Check sheet for the modelled part. Datum: model origin and axes. Units: mm. Face numbers are marked on the shaded views. A direction names the side the tool comes from. Give positions to 0.01 mm unless a question says otherwise; leave off trailing zeros. Order: outer loops, then holes, each group sorted by start corner. A loop starts at its lowest first (then second) coordinate and runs counter-clockwise, first axis right, second up.
Item 1: Sectioned sample at A-A on z = -4. Record the boundary of the cut face in (x, y), and give its area (3 significant figures).
Item 2: Sectioned sample at B-B on x = 0. Record the boundary of the cut face in (y, z).
Item 3: Gauge pin test, flat ends, axial feed: P1, Ø1.8, axis at x = 0, y = 5, coming from the +Z side; P2, Ø0.9, axis at x = -15, y = -3, coming from the -Z side; P3, Ø1.5, axis at y = 2.5, z = -1, coming from the -X side; P4, Ø1.8, axis at x = 15, y = -3, coming from the -Z side. Record the tip position at first contact, or that the pin passes through.
Item 4: Release check for a two-part mould opening along Y. For the marked faces 1, 2 and 3 record: released by +Y, released by -Y, zero draft, split by the parting line, or undercut.
Item 5: Sectioned sample at C-C on z = -2. Record the boundary of the cut face in (x, y), and give its area (3 significant figures).
Item 6: Access from +Z, -Z, +X, -X, +Y, -Y to the whole of each face (thin tool, end or side, straight path). Record for the marked faces 4, 5 and 6.
Item 7: Material ranges on line 1 along Y through (x, z) = (-15, -4.15); line 2 along X through (y, z) = (-3.25, -5.5); line 3 along Y through (x, z) = (15, -6.25), recorded low to high.
Item 8: Sectioned sample at D-D on y = 3. Record the boundary of the cut face in (x, z), and give its area (3 significant figures).
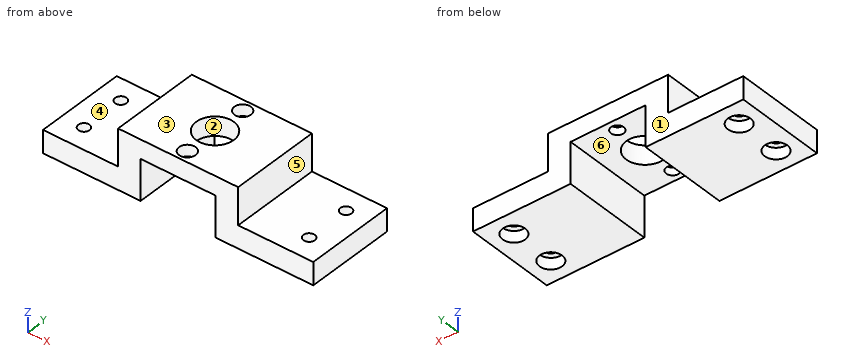
from build123d import *

# Parameters (mm, degrees)
SKETCH_1_W          = 10
SKETCH_1_H          = 12
SKETCH_1_R          = 0.85
SKETCH_1_R_2        = 2.5
EXTRUDE_1_DEPTH     = 1.25
CUT_EXTRUDE_START   = 1.25
SKETCH_1_6_R        = 1.1
CUT_EXTRUDE_1_DEPTH = 1.5
SKETCH_2_W          = 3
SKETCH_2_H          = 12
EXTRUDE_2_DEPTH     = 7.9
SKETCH_3_W          = 10
SKETCH_3_H          = 3
EXTRUDE_3_DEPTH     = 12
SKETCH_4_R          = 0.75
CUT_EXTRUDE_2_DEPTH = 21.552615405
SKETCH_4_3_R        = 1.5
CUT_EXTRUDE_3_DEPTH = 1.5


with BuildPart() as part:
    # 草图1 → 凸台-拉伸1 (new, symmetric)
    with BuildSketch(Plane.XY):
        Rectangle(SKETCH_1_W, SKETCH_1_H)
        with Locations((0, 4.5)):
            Circle(SKETCH_1_R, mode=Mode.SUBTRACT)
        with Locations((0, -4.5)):
            Circle(SKETCH_1_R, mode=Mode.SUBTRACT)
        Circle(SKETCH_1_R_2, mode=Mode.SUBTRACT)
    extrude(amount=EXTRUDE_1_DEPTH, both=True)

    # 草图1<6> → 切除-拉伸1 (cut)
    with BuildSketch(Plane.XY.offset(CUT_EXTRUDE_START)):
        with Locations((0, 4.5)):
            Circle(SKETCH_1_6_R)
        with Locations((0, -4.5)):
            Circle(SKETCH_1_6_R)
    extrude(amount=-CUT_EXTRUDE_1_DEPTH, mode=Mode.SUBTRACT)

    # 草图2 → 凸台-拉伸2 (add)
    with BuildSketch(Plane.XY.offset(1.25)):
        with Locations((6.5, 0)):
            Rectangle(SKETCH_2_W, SKETCH_2_H)
        with Locations((-6.5, 0)):
            Rectangle(SKETCH_2_W, SKETCH_2_H)
    extrude(amount=-EXTRUDE_2_DEPTH)

    # 草图3 → 凸台-拉伸3 (add)
    with BuildSketch(Plane(origin=(0, 6, 0), x_dir=(1, 0, 0), z_dir=(0, 1, 0))):
        with Locations((-13, 5.15)):
            Rectangle(SKETCH_3_W, SKETCH_3_H)
        with Locations((13, 5.15)):
            Rectangle(SKETCH_3_W, SKETCH_3_H)
    extrude(amount=-EXTRUDE_3_DEPTH)

    # 草图4 → 切除-拉伸2 (cut, through all)
    with BuildSketch(Plane(origin=(0, 0, -6.65), x_dir=(-1, 0, 0), z_dir=(0, 0, -1))):
        with Locations((15, -3)):
            Circle(SKETCH_4_R)
        with Locations((15, 3)):
            Circle(SKETCH_4_R)
        with Locations((-15, -3)):
            Circle(SKETCH_4_R)
        with Locations((-15, 3)):
            Circle(SKETCH_4_R)
    extrude(amount=-CUT_EXTRUDE_2_DEPTH, mode=Mode.SUBTRACT)

    # 草图4<3> → 切除-拉伸3 (cut)
    with BuildSketch(Plane(origin=(0, 0, -6.65), x_dir=(-1, 0, 0), z_dir=(0, 0, -1))):
        with Locations((15, 3)):
            Circle(SKETCH_4_3_R)
        with Locations((15, -3)):
            Circle(SKETCH_4_3_R)
        with Locations((-15, 3)):
            Circle(SKETCH_4_3_R)
        with Locations((-15, -3)):
            Circle(SKETCH_4_3_R)
    extrude(amount=-CUT_EXTRUDE_3_DEPTH, mode=Mode.SUBTRACT)


solid = part.part
Report:
1. outline: (-18, -6) - (-5, -6) - (-5, 6) - (-18, 6) - close; (5, -6) - (18, -6) - (18, 6) - (5, 6) - close; hole circle Ø1.5 at (-15, -3); hole circle Ø1.5 at (-15, 3); hole circle Ø1.5 at (15, -3); hole circle Ø1.5 at (15, 3)
1. area: 305 mm2
2. outline: (-6, -1.25) - (-5.35, -1.25) - (-5.35, -0.25) - (-5.6, -0.25) - (-5.6, 1.25) - (-6, 1.25) - close; (-3.65, -1.25) - (-2.5, -1.25) - (-2.5, 1.25) - (-3.4, 1.25) - (-3.4, -0.25) - (-3.65, -0.25) - close; (2.5, -1.25) - (3.65, -1.25) - (3.65, -0.25) - (3.4, -0.25) - (3.4, 1.25) - (2.5, 1.25) - close; (5.35, -1.25) - (6, -1.25) - (6, 1.25) - (5.6, 1.25) - (5.6, -0.25) - (5.35, -0.25) - close
3. P1: stops at z = 1.25
3. P2: passes through
3. P3: stops at x = -8
3. P4: stops at z = -5.15
4. face 1: released by +Y
4. face 2: undercut
4. face 3: zero draft
5. outline: (-8, -6) - (-5, -6) - (-5, 6) - (-8, 6) - close; (5, -6) - (8, -6) - (8, 6) - (5, 6) - close
5. area: 72.0 mm2
6. face 4: +Z, -X, +Y, -Y
6. face 5: +Z, +X, +Y, -Y
6. face 6: -Z, +Y, -Y
7. line 1: y = -6 to -3.75, -2.25 to 2.25, 3.75 to 6
7. line 2: x = -18 to -16.48, -13.52 to -5, 5 to 13.52, 16.48 to 18
7. line 3: y = -6 to -4.5, -1.5 to 1.5, 4.5 to 6
8. outline: (-18, -6.65) - (-16.5, -6.65) - (-16.5, -5.15) - (-15.75, -5.15) - (-15.75, -3.65) - (-18, -3.65) - close; (-14.25, -5.15) - (-13.5, -5.15) - (-13.5, -6.65) - (-5, -6.65) - (-5, -1.25) - (5, -1.25) - (5, -6.65) - (13.5, -6.65) - (13.5, -5.15) - (14.25, -5.15) - (14.25, -3.65) - (8, -3.65) - (8, 1.25) - (-8, 1.25) - (-8, -3.65) - (-14.25, -3.65) - close; (15.75, -5.15) - (16.5, -5.15) - (16.5, -6.65) - (18, -6.65) - (18, -3.65) - (15.75, -3.65) - close
8. area: 119 mm2
